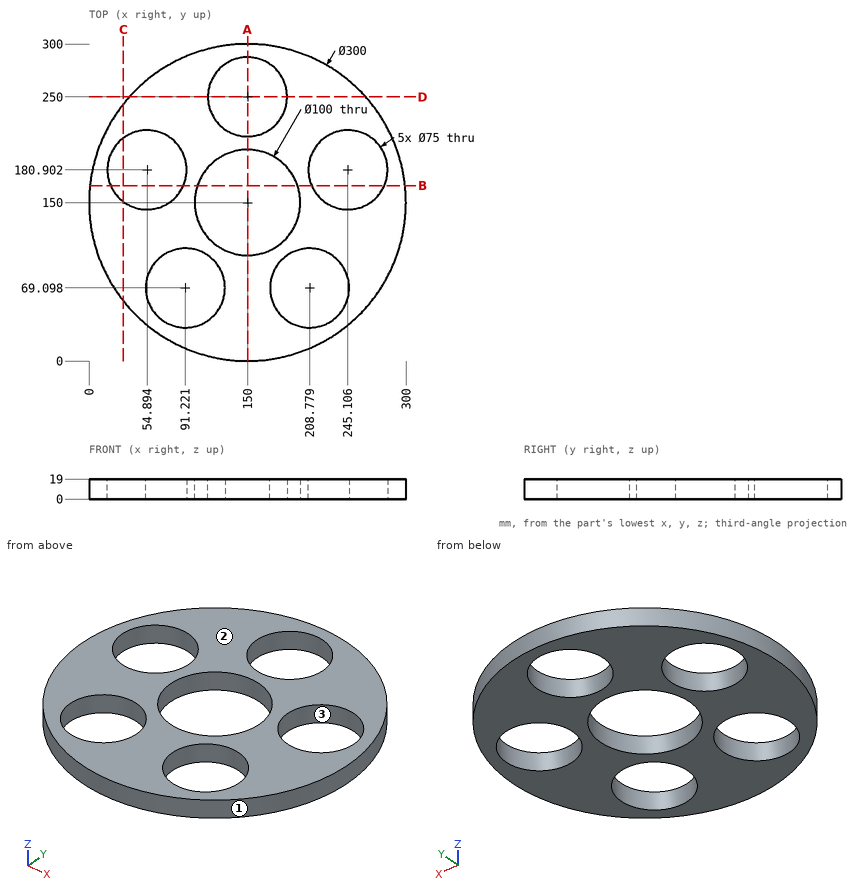
Source: three-view drawing plus pictorial views. Frame: mm from the lowest corner of the part. Round coordinates to 2 decimals unless told otherwise and drop trailing zeros. Loops run counter-clockwise (first coordinate to the right, second up) from the corner with the lowest first, then second, coordinate; pieces in that order, holes last.
Q1. Section B-B, the plane y = 166. Return loops of the section in (x, z) (1 decimal).
Q2. Section C-C, the plane x = 32.5. Return loops of the section in (y, z).
Q3. Section D-D, the plane y = 250. Return loops of the section in (x, z), plus the area to 3 significant figures.
Q4. Section A-A, the plane x = 150. Return loops of the section in (y, z).
Q5. Mould query, pull axis Y, two halves, no side actions, for the marked faces 1, 2 and 3. Classes: pulls with the +Y half, pulls with the -Y half, needs draft (parallel to the pull), parting line crosses it, or undercut.
Q6. First-contact query: P1, Ø2, axis at y = 239.5, z = 14, coming from the -X side; P2, Ø1.5, axis at x = 61, z = 9.5, coming from the -Y side; P3, Ø8, axis at x = 80.5, z = 3, coming from the -Y side. Flat tips, straight axial feed; report the tip coordinate or a pass-through.
Q7. Ray query, line 1 (Y direction, x = 150, z = 15.25); line 2 (Y direction, x = 80, z = 8.5) (1 decimal); line 3 (X direction, y = 187, z = 17.25) (1 decimal). Return the intervals inside material, ascending.
Solutions:
1. outline: (0.9, 0) - (20.5, 0) - (20.5, 19) - (0.9, 19) - close; (89.3, 0) - (102.6, 0) - (102.6, 19) - (89.3, 19) - close; (197.4, 0) - (210.7, 0) - (210.7, 19) - (197.4, 19) - close; (279.5, 0) - (299.1, 0) - (299.1, 19) - (279.5, 19) - close
2. outline: (56.76, 0) - (150.82, 0) - (150.82, 19) - (56.76, 19) - close; (210.98, 0) - (243.24, 0) - (243.24, 19) - (210.98, 19) - close
3. outline: (38.2, 0) - (112.5, 0) - (112.5, 19) - (38.2, 19) - close; (187.5, 0) - (261.8, 0) - (261.8, 19) - (187.5, 19) - close
3. area: 2,820 mm2
4. outline: (0, 0) - (100, 0) - (100, 19) - (0, 19) - close; (200, 0) - (212.5, 0) - (212.5, 19) - (200, 19) - close; (287.5, 0) - (300, 0) - (300, 19) - (287.5, 19) - close
5. face 1: parting line crosses it
5. face 2: needs draft
5. face 3: undercut
6. P1: stops at x = 28.89
6. P2: stops at y = 28.71
6. P3: stops at y = 15.06
7. line 1: y = 0 to 100, 200 to 212.5, 287.5 to 300
7. line 2: y = 17.3 to 33.3, 104.9 to 153, 208.8 to 282.7
7. line 3: x = 4.6 to 17.9, 91.9 to 116.4, 183.6 to 208.1, 282.1 to 295.4
